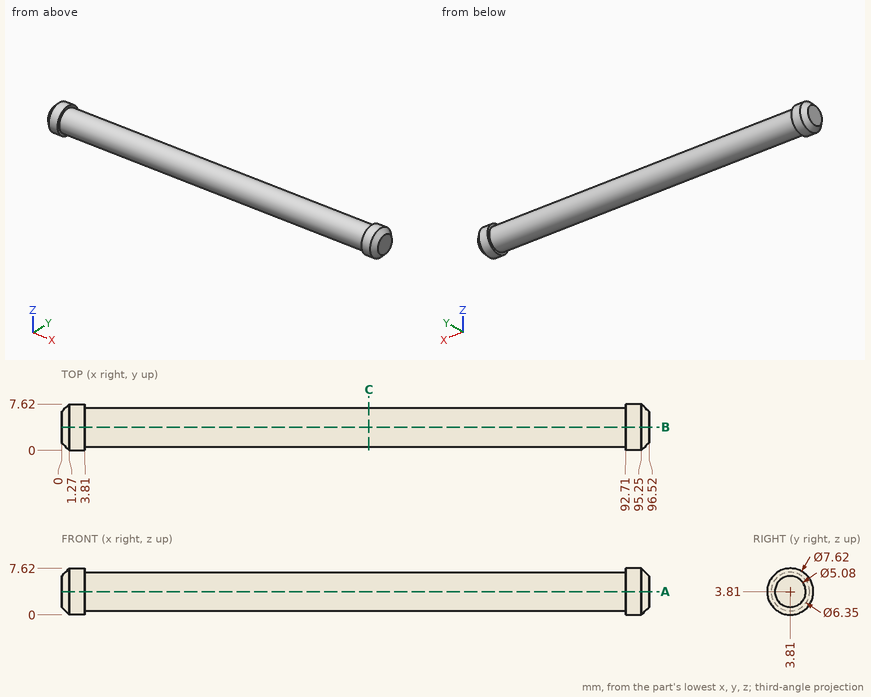
Geometry check sheet. Reference: drawing and pictorial views, mm from the part's lowest x, y, z. Coordinates: 2 decimals unless noted, no trailing zeros. Order: outer loops, then holes, each group sorted by start corner. A loop starts at its lowest first (then second) coordinate and runs counter-clockwise, first axis right, second up.
1. Go/stop test with flat-tipped pins: pin 1 Ø2 at (x, y) = (81, 4) entering from -Z (3 decimals); pin 2 Ø2 at (x, y) = (39.5, 3.5) entering from +Z (3 decimals). Record where each tip stops, or that it passes through.
Results found:
pin 1: stops at z = 0.635
pin 2: stops at z = 6.985
2. Sectioned sample at A-A, the plane z = 3.81. Record the cut outline in (x, y) (3 decimals).
Results found:
outline: (0, 1.27) - (1.27, 0) - (3.81, 0) - (3.81, 0.635) - (92.71, 0.635) - (92.71, 0) - (95.25, 0) - (96.52, 1.27) - (96.52, 6.35) - (95.25, 7.62) - (92.71, 7.62) - (92.71, 6.985) - (3.81, 6.985) - (3.81, 7.62) - (1.27, 7.62) - (0, 6.35) - close
3. Scan lines: line 1 (Y direction, x = 82.5, z = 3.75); line 2 (X direction, y = 0.5, z = 3.5); line 3 (Y direction, x = 29, z = 5.75). Record each from-to range of solid material in increasing order.
Results found:
line 1: y = 0.64 to 6.98
line 2: x = 0.78 to 3.81, 92.71 to 95.74
line 3: y = 1.3 to 6.32
4. Sectioned sample at C-C, the plane x = 50.5. Record the cut outline in (y, z) (3 decimals), and give its area (3 significant figures).
Results found:
outline: circle Ø6.35 at (3.81, 3.81)
area: 31.7 mm2
